Answer from the drawing. Dimensions are ordinates in mm from the lowest x, y and z of the part. A direction names the side the tool comes from. Give positions to 0.01 mm unless a question says otherwise; leave off trailing zeros. Order: outer loops, then holes, each group sorted by start corner. A loop starts at its lowest first (then second) coordinate and runs counter-clockwise, first axis right, second up. Notation, with made-up numbers: (-21, 66) - (22, 66) arc R21 cw to (22, 72) - close; hole circle Ø6 at (-32, -18). An arc over 180 degrees is marked (long way). Answer in a Markdown table with one row per item. Add a question column.
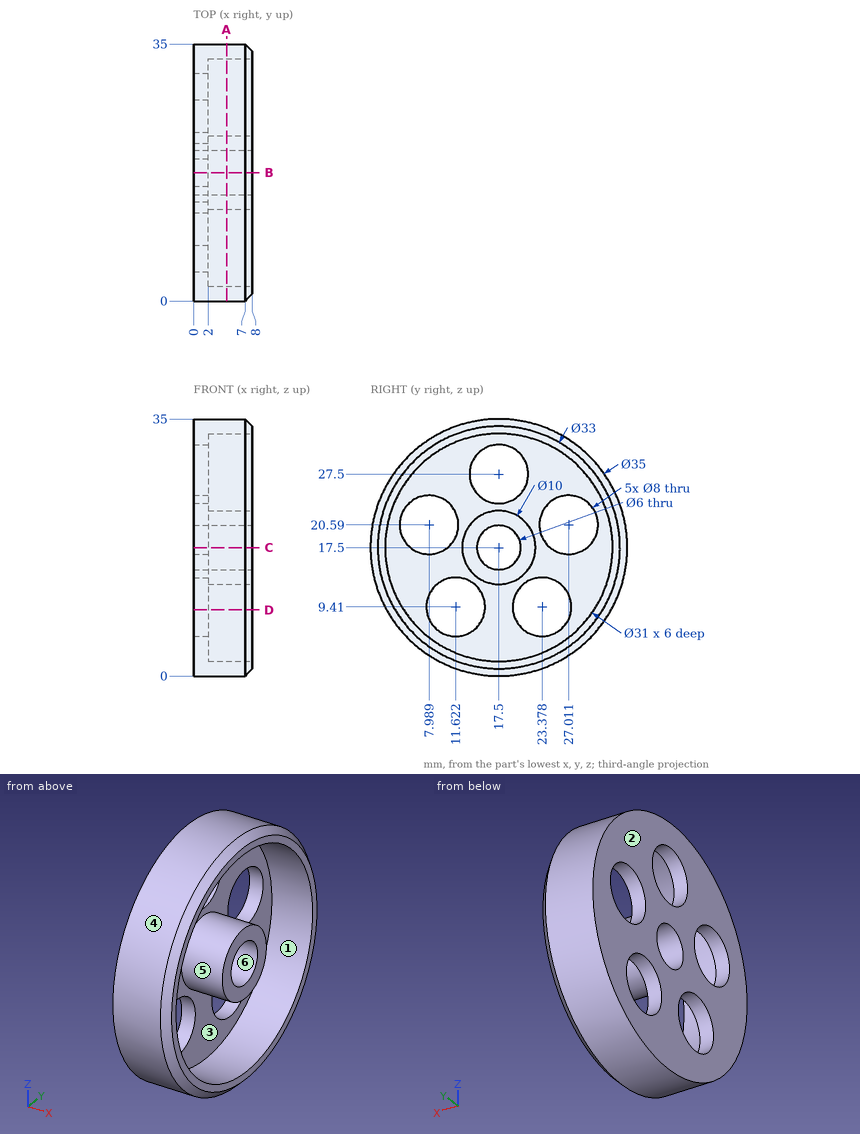
(1) Each of these flat-tipped pins is pushed along its axis until it touches: P1, Ø9, axis at y = 23.38, z = 9.41, coming from the +X side; P2, Ø5.5, axis at y = 17.5, z = 17.5, coming from the +X side; P3, Ø10, axis at y = 29, z = 30, coming from the +X side; P4, Ø1.5, axis at x = 6, z = 30, coming from the -Y side. Where does it stop, or does it pass through?
(2) Find section D-D, the plane z = 9. Give the number of separate pieces and of enclosed holes in the cut face.
(3) Find section B-B, the plane y = 17.5. Write down the section's boundary in (x, z).
(4) Find section A-A, the plane x = 4.5. Write down the section's boundary in (y, z).
(5) The mould has two halves that part along Y. Classify the marked faces 1, 2, 3 and 4: +Y half, -Y half, draft (parallel to the pull), parting line (faces both ways), or undercut.
(6) For the marked faces 5 and 6, determine the directions among +Z, -Z, +X, -X, +Y, -Y from which every point of the face is accessible in a straight line to the end or side of a thin tool.
(7) Find section C-C, the plane z = 17.5. Write down the section's boundary in (x, y).
(8) Straight lines are drawn through the part: line 1 (Z direction, x = 1.2, y = 17.5); line 2 (Z direction, x = 2.25, y = 17.5). For each, find the intervals that lie inside material, in ascending order.
Answer key:
| question | item | result |
|---|---|---|
| 1 | P1 | x = 2 |
| 1 | P2 | through |
| 1 | P3 | x = 8 |
| 1 | P4 | y = 4.53 |
| 2 | separate pieces | 3 |
| 2 | enclosed holes | 0 |
| 3 | outline | (0, 0) - (7, 0) - (8, 1) - (8, 2) - (2, 2) - (2, 12.5) - (8, 12.5) - (8, 14.5) - (0, 14.5) - close; (0, 20.5) - (8, 20.5) - (8, 22.5) - (2, 22.5) - (2, 23.5) - (0, 23.5) - close; (0, 31.5) - (2, 31.5) - (2, 33) - (8, 33) - (8, 34) - (7, 35) - (0, 35) - close |
| 4 | outline | circle Ø35 at (17.5, 17.5); circle Ø10 at (17.5, 17.5); hole circle Ø31 at (17.5, 17.5); hole circle Ø6 at (17.5, 17.5) |
| 5 | face 1 | undercut |
| 5 | face 2 | draft |
| 5 | face 3 | undercut |
| 5 | face 4 | parting line |
| 6 | face 5 | +X |
| 6 | face 6 | +X, -X |
| 7 | outline | (0, 0) - (7, 0) - (8, 1) - (8, 2) - (2, 2) - (2, 5.45) - (0, 5.45) - close; (0, 10.53) - (2, 10.53) - (2, 12.5) - (8, 12.5) - (8, 14.5) - (0, 14.5) - close; (0, 20.5) - (8, 20.5) - (8, 22.5) - (2, 22.5) - (2, 24.47) - (0, 24.47) - close; (0, 29.55) - (2, 29.55) - (2, 33) - (8, 33) - (8, 34) - (7, 35) - (0, 35) - close |
| 8 | line 1 | 0 to 14.5, 20.5 to 23.5, 31.5 to 35 |
| 8 | line 2 | 0 to 2, 12.5 to 14.5, 20.5 to 22.5, 33 to 35 |
